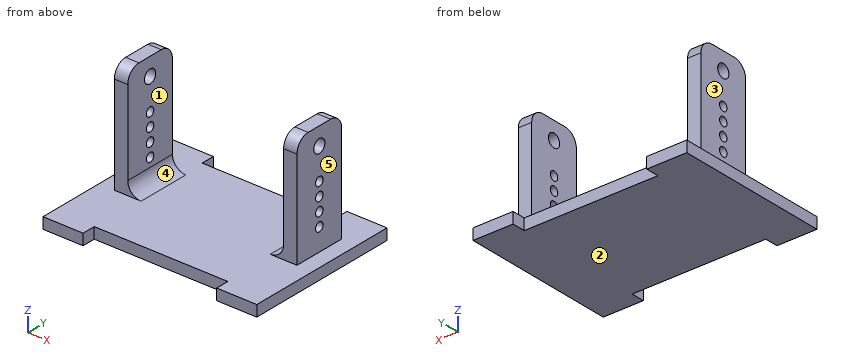
```python
from build123d import *

# Parameters (mm, degrees)
BOSS_EXTRU_1_DEPTH      = 2.5
ESQUISSE2_W             = 3
ESQUISSE2_H             = 12
BOSS_EXTRU_2_DEPTH      = 25
ESQUISSE3_R             = 1
ESQUISSE3_R_2           = 1.5
ENL_V_MAT_EXTRU_1_DEPTH = 50
CONG_1_R                = 3
CONG_2_R                = 3


with BuildPart() as part:
    # Esquisse1 → Boss.-Extru.1 (new body)
    with BuildSketch(Plane.XY):
        Polygon((39, 35), (48, 35), (48, 0), (39, 0), (39, 3), (9, 3), (9, 0), (0, 0), (0, 35), (9, 35), (9, 32), (39, 32), align=None)
    extrude(amount=BOSS_EXTRU_1_DEPTH)

    # Esquisse2 → Boss.-Extru.2 (add)
    with BuildSketch(Plane.XY.offset(2.5)):
        with Locations((5, 21)):
            Rectangle(ESQUISSE2_W, ESQUISSE2_H)
        with Locations((43, 21)):
            Rectangle(ESQUISSE2_W, ESQUISSE2_H)
    extrude(amount=BOSS_EXTRU_2_DEPTH)

    # Esquisse3 → Enlèv. mat.-Extru.1 (cut)
    with BuildSketch(Plane(origin=(44.5, 0, 0), x_dir=(0, 0, -1), z_dir=(1, 0, 0))):
        with Locations((-7.5, 21)):
            Circle(ESQUISSE3_R)
        with Locations((-10.5, 21)):
            Circle(ESQUISSE3_R)
        with Locations((-13.5, 21)):
            Circle(ESQUISSE3_R)
        with Locations((-16.5, 21)):
            Circle(ESQUISSE3_R)
        with Locations((-23.5, 21)):
            Circle(ESQUISSE3_R_2)
    extrude(amount=-ENL_V_MAT_EXTRU_1_DEPTH, mode=Mode.SUBTRACT)

    # Congé1
    cong_1_edges = [part.edges().sort_by_distance(p)[0] for p in [
        (5, 15, 27.5),
        (5, 27, 27.5),
        (43, 15, 27.5),
        (43, 27, 27.5),
    ]]
    fillet(cong_1_edges, radius=CONG_1_R)

    # Congé2
    cong_2_edges = [part.edges().sort_by_distance(p)[0] for p in [
        (6.5, 21, 2.5),
        (41.5, 21, 2.5),
    ]]
    fillet(cong_2_edges, radius=CONG_2_R)


solid = part.part
```
The model under review builds one solid part; all positions refer to its coordinate system, in mm. Face numbers are marked on the shaded views. A direction names the side the tool comes from. Round coordinates to 2 decimals unless told otherwise and drop trailing zeros. Loops run counter-clockwise (first coordinate to the right, second up) from the corner with the lowest first, then second, coordinate; pieces in that order, holes last.
Item 1: For the marked faces 1 and 2, list the 3-axis set-ups (+Z, -Z, +X, -X, +Y, -Y) from which the entire face can be reached by the end or side of a thin tool; tool diameter is ignored.
Determined:
face 1: +Z, +Y, -Y
face 2: -Z, +X, -X, +Y, -Y
Item 2: For line 1 (Y direction, x = 5.05, z = 16.5); line 2 (X direction, y = 19.5, z = 19.25); line 3 (Z direction, x = 21.5, y = 21.5), list the stretches that pass through material, from the lowest coordinate up.
Determined:
line 1: y = 15 to 20, 22 to 27
line 2: x = 3.5 to 6.5, 41.5 to 44.5
line 3: z = 0 to 2.5
Item 3: Mouldability with a two-part tool opening along X and no side actions: class the marked faces 3, 4 and 5 as released by +X, released by -X, zero draft, split by the parting line, or undercut.
Determined:
face 3: released by -X
face 4: undercut
face 5: released by +X
Item 4: Take a section at C-C (z = 4.25). Write out the cut boundary in (x, y).
Determined:
outline: (3.5, 15) - (6.77, 15) - (6.77, 27) - (3.5, 27) - close; (41.23, 15) - (44.5, 15) - (44.5, 27) - (41.23, 27) - close
Item 5: Clearance check with flat-ended pins moving along their axes: pin 1 Ø1.2 at (x, z) = (31, 1.5) entering from +Y; pin 2 Ø12 at (y, z) = (20, 18.5) entering from +X; pin 3 Ø13 at (y, z) = (20.5, 14) entering from -X. State where each tip first meets the part, or that it passes through.
Determined:
pin 1: stops at y = 32
pin 2: stops at x = 44.5
pin 3: stops at x = 3.5
Item 6: Take a section at A-A (z = 7.5). Write out the cut boundary in (x, y).
Determined:
outline: (3.5, 15) - (6.5, 15) - (6.5, 20) - (3.5, 20) - close; (3.5, 22) - (6.5, 22) - (6.5, 27) - (3.5, 27) - close; (41.5, 15) - (44.5, 15) - (44.5, 20) - (41.5, 20) - close; (41.5, 22) - (44.5, 22) - (44.5, 27) - (41.5, 27) - close
Item 7: Take a section at D-D (y = 21). Give the number of separate pieces and of enclosed holes in the cut face, then the cut area to 3 significant figures.
Determined:
separate pieces: 11
enclosed holes: 0
area: 208 mm2
Item 8: Take a section at B-B (x = 4.5). Write out the cut boundary in (y, z), then the cut area to 3 significant figures.
Determined:
outline: (0, 0) - (35, 0) - (35, 2.5) - (27, 2.5) - (27, 24.5) arc R3 ccw to (24, 27.5) - (18, 27.5) arc R3 ccw to (15, 24.5) - (15, 2.5) - (0, 2.5) - close; hole circle Ø3 at (21, 23.5); hole circle Ø2 at (21, 7.5); hole circle Ø2 at (21, 10.5); hole circle Ø2 at (21, 13.5); hole circle Ø2 at (21, 16.5)
area: 364 mm2
